```python
from build123d import *

# Parameters (mm, degrees)
SKETCH1_R           = 1.5875
BOSS_EXTRUDE1_DEPTH = 9.525
SKETCH2_W           = 6.35
SKETCH2_H           = 3.175
BOSS_EXTRUDE2_DEPTH = 6.35
SKETCH3_R           = 1.5875
CUT_EXTRUDE1_DEPTH  = 17.497783942
FILLET1_R           = 3.175


with BuildPart() as part:
    # Sketch1 → Boss-Extrude1 (new body)
    with BuildSketch(Plane(origin=(0, 0, 0), x_dir=(1, 0, 0), z_dir=(0, 1, 0))):
        with Locations(Location((0, 0, 0), (0, 0, 90))):
            Circle(SKETCH1_R)
    boss_extrude1 = extrude(amount=BOSS_EXTRUDE1_DEPTH)

    # Sketch2 → Boss-Extrude2 (add)
    with BuildSketch(Plane(origin=(0, 9.525, 0), x_dir=(1, 0, 0), z_dir=(0, 1, 0))):
        Rectangle(SKETCH2_W, SKETCH2_H)
    boss_extrude2 = extrude(amount=BOSS_EXTRUDE2_DEPTH)

    # Sketch3 → Cut-Extrude1 (cut, through all)
    with BuildSketch(Plane(origin=(0, 0, -1.5875), x_dir=(-1, 0, 0), z_dir=(0, 0, -1))):
        with Locations((0, 12.7)):
            Circle(SKETCH3_R)
    cut_extrude1 = extrude(amount=-CUT_EXTRUDE1_DEPTH, mode=Mode.SUBTRACT)

    # Mirror1: Boss-Extrude1, Boss-Extrude2, Cut-Extrude1 across plane
    add(boss_extrude1.mirror(Plane.ZX))
    add(boss_extrude2.mirror(Plane.ZX))
    add(cut_extrude1.mirror(Plane.ZX), mode=Mode.SUBTRACT)

    # Fillet1
    fillet1_edges = [part.edges().sort_by_distance(p)[0] for p in [
        (-3.175, -15.875, 0),
        (3.175, -15.875, 0),
        (-3.175, 15.875, 0),
        (3.175, 15.875, 0),
    ]]
    fillet(fillet1_edges, radius=FILLET1_R - 0.0001)  # a hair under: the kernel refuses the full size


solid = part.part
```
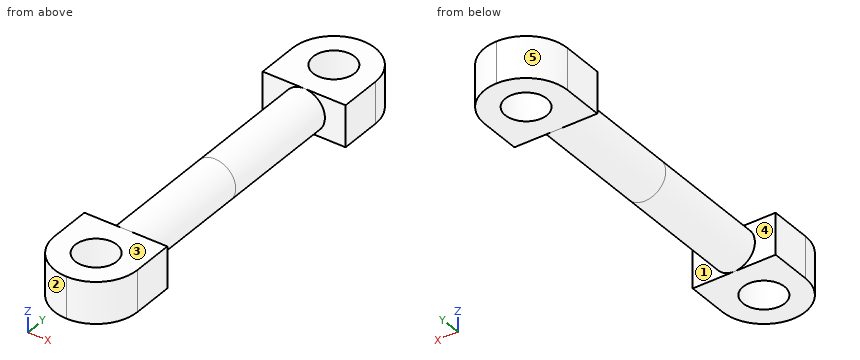
Design review of the part built by this model. Coordinates are the model's own, in mm. Face numbers are marked on the shaded views. A direction names the side the tool comes from. Coordinates: 2 decimals unless noted, no trailing zeros. Write each loop counter-clockwise with the first axis right and the second up, starting at its lowest first coordinate (ties: lowest second). Pieces come first, ordered by that corner, then holes.
1) Add section B-B (x = 2.5). Write out the cut boundary in (y, z) (1 decimal), plus the area to 3 significant figures.
2) Machinability: for the marked faces 1 and 2, which of the approach directions +Z, -Z, +X, -X, +Y, -Y give a long, thin tool a straight path to every point of the face, cutting with its end or side? Answer none if there is none.
3) Insertion check: pin 1 (3 mm diameter, centred on x = 0, y = 12.7, fed in from +Z); pin 2 (1 mm diameter, centred on x = 1.5, z = 1, fed in from -Y); pin 3 (1 mm diameter, centred on x = 2, z = 0.5, fed in from +Y); pin 4 (1.6 mm diameter, centred on x = -2, z = 0, fed in from +Y). Each pin has a flat end and moves straight along its axis. Give the tip position at first contact, or say it passes through.
4) To check wall thickness, follow L1, parallel to Y at x = 0, z = -0.55 (1 decimal); L2, parallel to X at y = -12.7, z = 0.6 (1 decimal); L3, parallel to Y at x = 1, z = -0.85. State the ranges of each line that lie inside material, in increasing order.
5) Add section C-C (y = 14). Write out the cut boundary in (x, z).
6) Mouldability with a two-part tool opening along Y and no side actions: class the marked faces 3, 4 and 5 as +Y half, -Y half, draft (parallel to the pull), parting line (faces both ways), or undercut.
7) Add section A-A (z = 0). State how many separate pieces and enclosed holes the cut face has, plus the area to 3 significant figures.
Check result:
1. outline: (-14.7, -1.6) - (-9.5, -1.6) - (-9.5, 1.6) - (-14.7, 1.6) - close; (9.5, -1.6) - (14.7, -1.6) - (14.7, 1.6) - (9.5, 1.6) - close
1. area: 32.6 mm2
2. face 1: +X
2. face 2: +Z, -Z, -X, -Y
3. pin 1: passes through
3. pin 2: stops at y = -15.71
3. pin 3: stops at y = 15.5
3. pin 4: stops at y = 15.64
4. L1: y = -15.9 to -14.3, -11.1 to 11.1, 14.3 to 15.9
4. L2: x = -3.2 to -1.6, 1.6 to 3.2
4. L3: y = -15.71 to -13.93, -11.47 to 11.47, 13.93 to 15.71
5. outline: (-2.9, -1.59) - (-0.91, -1.59) - (-0.91, 1.59) - (-2.9, 1.59) - close; (0.91, -1.59) - (2.9, -1.59) - (2.9, 1.59) - (0.91, 1.59) - close
6. face 3: draft
6. face 4: undercut
6. face 5: +Y half
7. separate pieces: 1
7. enclosed holes: 2
7. area: 117 mm2
